```python
from build123d import *

# Parameters (mm, degrees)
F0_R          = 5
F1_DEPTH      = 2
F2_R          = 3.4
F3_DEPTH      = 15
F5_R          = 3.75
F5_R_2        = 1.5
F6_DEPTH      = 2
F7_R          = 1.5
F8_DEPTH      = 25
F8_DEPTH_BACK = 25
F9_SIZE       = 2
F10_R         = 3.5
F10_R_2       = 3
F11_DEPTH     = 5


with BuildPart() as f1:
    # F0 (on Front) → F1 (new body)
    with BuildSketch(Plane.XZ):
        Circle(F0_R)
    extrude(amount=F1_DEPTH)

    # F2 (on face) → F3 (join)
    with BuildSketch(Plane.XZ.offset(2)):
        Circle(F2_R)
    extrude(amount=F3_DEPTH)

    # F5 (on offset) → F6 (cut)
    with BuildSketch(Plane.XZ.offset(12)):
        Circle(F5_R)
        Circle(F5_R_2, mode=Mode.SUBTRACT)
    extrude(amount=F6_DEPTH, mode=Mode.SUBTRACT)

    # F7 (on Right) → F8 (cut, two sides)
    with BuildSketch(Plane.YZ) as f8_sk:
        with Locations((-8, 0)):
            Circle(F7_R)
    extrude(amount=F8_DEPTH, mode=Mode.SUBTRACT)
    extrude(f8_sk.sketch, amount=-F8_DEPTH_BACK, mode=Mode.SUBTRACT)

    # F9
    f9_edges = [f1.edges().sort_by_distance(p)[0] for p in [
        (-3.4, -17, 0),
    ]]
    chamfer(f9_edges, length=F9_SIZE)

    # F10 (on face) → F11 (cut)
    with BuildSketch(Plane.XZ.offset(17)):
        Circle(F10_R)
        Circle(F10_R_2, mode=Mode.SUBTRACT)
    extrude(amount=-F11_DEPTH, mode=Mode.SUBTRACT)


solid = f1.part
```
Read the model definition and answer for the solid it produces. Units are mm, in the model's axes. A direction names the side the tool comes from. Give positions to 0.01 mm unless a question says otherwise; leave off trailing zeros. Order: outer loops, then holes, each group sorted by start corner. A loop starts at its lowest first (then second) coordinate and runs counter-clockwise, first axis right, second up. Notation, with made-up numbers: (-34.75, 71) -> (-23.75, 71) arc R23 cw to (-23.75, 105) -> close; hole circle Ø1 at (-19, -27.75). An arc over 180 degrees is marked (long way). One line per item, written item: value. Start each with the question number.
(1) Flat-ended cylindrical pins translate along their axes: P1, Ø2.5, axis at y = -8, z = 0, coming from the -X side; P2, Ø1, axis at y = -6.5, z = 2.5, coming from the -X side; P3, Ø1.5, axis at x = -3, y = -12.5, coming from the -Z side; P4, Ø5, axis at y = -8, z = 0, coming from the +X side. Find the tip coordinate at first contact, or state that the pin passes through.
(2) The part is cut by section B-B (x = -2.5). State how many separate pieces and enclosed holes the cut face has, and give its area (3 significant figures).
(3) The part is cut by section C-C (y = -8). Determine the outline of the cut face in (x, z), and give its area (3 significant figures).
(4) Straight lines are drawn through the part: L1, parallel to Y at x = 2.25, z = 1; L2, parallel to Y at x = 2.4, z = 0; L3, parallel to Y at x = -2.25, z = -2.75. For each, find the intervals that lie inside material, in ascending order.
(5) The part is cut by section A-A (z = 0). Determine the outline of the cut face in (x, y), and give its area (3 significant figures).
(6) For a pull along Y with two mould halves and no side action, classify faces 1 (the cylindrical face through (-1.08, -0.99, -4.88)), 2 (the flat face through (0, 0, 0)), 3 (the flat face through (1.5, -12, -0.7)) as released by +Y, released by -Y, zero draft, split by the parting line, or undercut.
(7) The part is cut by section D-D (y = -5). Determine the outline of the cut face in (x, z), and give its area (3 significant figures).
(8) A tool of negligible diameter and unlimited length cuts with its end or side. For faces 4 (the flat face through (1.3, -14, -1.3)), 5 (the flat face through (0, -17, 0)), 6 (the cylindrical face through (1.6, -6.9, -3)), from which of +Z, -Z, +X, -X, +Y, -Y can it reach the whole face along a straight path? Write none if from no direction.
Taken from the geometry:
1. P1: through
1. P2: x = -2.75
1. P3: z = -2.37
1. P4: x = 3.4
2. separate pieces: 2
2. enclosed holes: 1
2. area: 62.1 mm^2
3. outline: (-3.05, -1.5) arc R3.4 ccw to (3.05, -1.5) -> close; (-3.05, 1.5) -> (3.05, 1.5) arc R3.4 ccw to start
3. area: 16.6 mm^2
4. L1: -15.94 to -14, -12 to -9.12, -6.88 to 0
4. L2: -16 to -14, -12 to -9.5, -6.5 to 0
4. L3: -2 to 0
5. outline: (-5, -2) -> (-3.4, -2) -> (-3.4, -6.5) -> (3.4, -6.5) -> (3.4, -2) -> (5, -2) -> (5, 0) -> (-5, 0) -> close; (-3.4, -12) -> (-1.5, -12) -> (-1.5, -14) -> (-3, -14) -> (-3, -15.4) -> (-1.4, -17) -> (1.4, -17) -> (3, -15.4) -> (3, -14) -> (1.5, -14) -> (1.5, -12) -> (3.4, -12) -> (3.4, -9.5) -> (-3.4, -9.5) -> close
5. area: 89.0 mm^2
6. face 1: zero draft
6. face 2: released by +Y
6. face 3: undercut
7. outline: circle Ø6.8 at (0, 0)
7. area: 36.3 mm^2
8. face 4: none
8. face 5: +Z, -Z, +X, -X, -Y
8. face 6: -Y
